Verification items for the finished model (mm, model axes). A direction names the side the tool comes from. Round coordinates to 2 decimals unless told otherwise and drop trailing zeros. Write each loop counter-clockwise with the first axis right and the second up, starting at its lowest first coordinate (ties: lowest second). Pieces come first, ordered by that corner, then holes. Notation, with made-up numbers: M 37,12 L 92,12 A30 ccw 92,48 Z; hole C 6,6 d3. An arc over 180 degrees is marked long. One line per question, with ' | ' between items.
Autodesk Inventor part; units mm, degrees
ref_plane "YZ Plane" through (0, 0, 0) normal (1, 0, 0) x (0, 1, 0)
ref_plane "XZ Plane" through (0, 0, 0) normal (0, 1, 0) x (-1, 0, 0)
ref_plane "XY Plane" through (0, 0, 0) normal (0, 0, 1) x (1, 0, 0)
sketch "Sketch1" plane through (0, 0, 0) normal (0, 1, 0) x (-1, 0, 0)
  line L0 (10, 38.5) -> (-10, 38.5)
  line L1 (-10, 38.5) -> (-10, -38.5)
  line L2 (-10, -38.5) -> (10, -38.5)
  line L3 (10, -38.5) -> (10, 38.5)
  line L4 (10, 38.5) -> (-10, -38.5) construction
  line L5 (-10, 38.5) -> (10, -38.5) construction
  point P0 (0, 0)
  dimension "d0" = 77
  dimension "d1" = 20
extrude "Extrusion1" add sketch "Sketch1" along normal blind 8
sketch "Sketch3" plane through (0, 8, 0) normal (0, 1, 0) x (1, 0, 0)
  circle A0 centre (0, -27.5) radius 2.5574
  circle A1 centre (0, 27.5) radius 2.6
  point P0 (0, 0)
  dimension "d8" = 5.2
  dimension "d9" = 55
  dimension "d10" = 27.5
extrude "Extrusion2" cut sketch "Sketch3" against normal blind 6
thread "Thread1"
thread "Thread2"
properties part number "Spannbacke(n)"
1. Mould release check, pull along X, two halves, no side actions. Record for faces 3 (the face through (-10, 4, -1)), 4 (the face through (-0.338, 5.042, -30.078)), 5 (the face through (0, 0, 1)): pulls with the +X half, pulls with the -X half, needs draft (parallel to the pull), parting line crosses it, or undercut.
Results:
face 3: pulls with the -X half | face 4: undercut | face 5: needs draft
2. Tool access check on faces 1 (the face through (0, 2, 27)), 2 (the face through (0, 4, 38.5)). Record the directions out of +Z, -Z, +X, -X, +Y, -Y that give a thin tool (end or side, any length) a straight path to the whole face; none if there is none.
Results:
face 1: +Y | face 2: +Z, +X, -X, +Y, -Y
3. Section check A-A, the plane y = 6.5. Record the cut outline in (x, z).
Results:
outline: M -10,-38.5 L 10,-38.5 L 10,38.5 L -10,38.5 Z; hole C 0,-27.5 d5.2; hole C 0,27.5 d5.11
4. Section check B-B, the plane z = 27.5. Record the cut outline in (x, y).
Results:
outline: M -10,0 L 10,0 L 10,8 L 2.56,8 L 2.56,2 L -2.56,2 L -2.56,8 L -10,8 Z
5. Thickness scan on line 1 (Z direction, x = 0, y = 4.2); line 2 (X direction, y = 6.15, z = 27.5); line 3 (Y direction, x = -0.5, z = -27.5). Record the ranges inside material, lowest first.
Results:
line 1: z = -38.5 to -30.1, -24.9 to 24.94, 30.06 to 38.5 | line 2: x = -10 to -2.56, 2.56 to 10 | line 3: y = 0 to 2
6. Section check C-C, the plane x = 0. Record the cut outline in (y, z).
Results:
outline: M 0,-38.5 L 8,-38.5 L 8,-30.1 L 2,-30.1 L 2,-24.9 L 8,-24.9 L 8,24.94 L 2,24.94 L 2,30.06 L 8,30.06 L 8,38.5 L 0,38.5 Z
7. Section check D-D, the plane z = -27.5. Record the cut outline in (x, y).
Results:
outline: M -10,0 L 10,0 L 10,8 L 2.6,8 L 2.6,2 L -2.6,2 L -2.6,8 L -10,8 Z
8. Go/stop test with a flat-tipped pin: P1, Ø4, axis at x = 0, z = 27.5, coming from the +Y side. Record where the tip stops, or that it passes through.
Results:
P1: stops at y = 2
